Read the model definition and answer for the solid it produces. Units are mm, in the model's axes. Coordinates: 2 decimals unless noted, no trailing zeros. Loops run counter-clockwise (first coordinate to the right, second up) from the corner with the lowest first, then second, coordinate; pieces in that order, holes last. Notation, with made-up numbers: M 72.25,-7.5 L 101.25,-7.5 A29 cw 101.25,12.5 Z; hole C -32.75,-21 d3. An arc over 180 degrees is marked long. One line per item, written item: value. Start each with the question number.
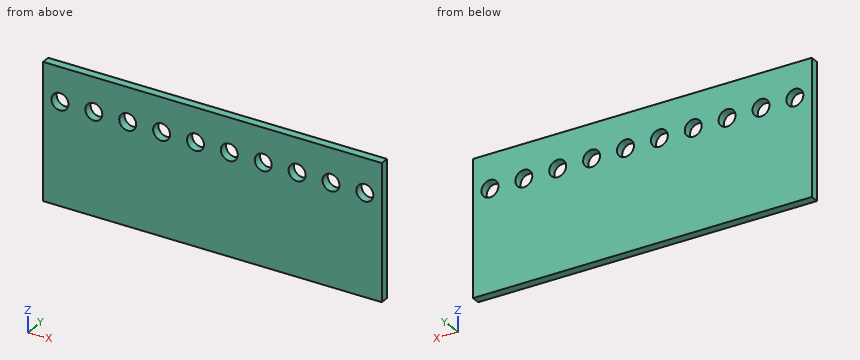
Autodesk Inventor part; units mm, degrees
ref_plane "YZ Plane" through (0, 0, 0) normal (1, 0, 0) x (0, 1, 0)
ref_plane "XZ Plane" through (0, 0, 0) normal (0, 1, 0) x (-1, 0, 0)
ref_plane "XY Plane" through (0, 0, 0) normal (0, 0, 1) x (1, 0, 0)
sketch "Sketch1" plane through (0, 0, 0) normal (0, 1, 0) x (-1, 0, 0)
  line L0 (127, 50.8) -> (-127, 50.8)
  line L1 (-127, 50.8) -> (-127, -50.8)
  line L2 (-127, -50.8) -> (127, -50.8)
  line L3 (127, -50.8) -> (127, 50.8)
  line L4 (127, 50.8) -> (-127, -50.8) construction
  line L5 (-127, 50.8) -> (127, -50.8) construction
  point P0 (0, 0)
  dimension "d3" = 101.6
  dimension "d13" = 254
extrude "Extrusion1" add sketch "Sketch1" against normal blind 6.35
sketch "Sketch3" plane through (0, 0, 0) normal (0, 1, 0) x (1, 0, 0)
  line L0 (-127, -50.8) -> (-127, 50.8) construction
  line L1 (-127, -25.4) -> (127, -25.4) construction
  line L2 (127, 50.8) -> (127, -50.8) construction
  line L3 (127, 50.8) -> (-127, 50.8) construction
  circle A0 centre (-114.3, -25.4) radius 6.35
  circle A1 centre (-88.9, -25.4) radius 6.35
  circle A2 centre (-63.5, -25.4) radius 6.35
  circle A3 centre (-38.1, -25.4) radius 6.35
  circle A4 centre (-12.7, -25.4) radius 6.35
  circle A5 centre (12.7, -25.4) radius 6.35
  circle A6 centre (38.1, -25.4) radius 6.35
  circle A7 centre (63.5, -25.4) radius 6.35
  circle A8 centre (88.9, -25.4) radius 6.35
  circle A9 centre (114.3, -25.4) radius 6.35
  point P0 (0, 0)
  dimension "d2" = 76.2
  dimension "d4" = 12.7
  dimension "d5" = 12.7
  dimension "d8" = 25.4
extrude "Extrusion2" cut sketch "Sketch3" against normal through all
properties part number "10-holes"
1) Consider line 1 along Z through (x, y) = (63.5, -5); line 2 along Z through (x, y) = (43, -2.5). Determine where each line is inside the solid, lowest interval first.
2) Section A-A (x = 63.5) is taken. Determine the outline of the cut face in (y, z), then the cut area to 3 significant figures.
3) Section B-B (y = -2) is taken. Count the separate pieces of the cut face and the enclosed holes in it, then the cut area to 3 significant figures.
4) A flat-ended cylindrical pin translates along its axis: pin 1 (7.5 mm diameter, centred on x = -12.7, z = 25.4, fed in from -Y). Find the tip coordinate at first contact, or state that the pin passes through.
Results found:
1. line 1: z = -50.8 to 19.05, 31.75 to 50.8
1. line 2: z = -50.8 to 21.36, 29.44 to 50.8
2. outline: M -6.35,-50.8 L 0,-50.8 L 0,19.05 L -6.35,19.05 Z; M -6.35,31.75 L 0,31.75 L 0,50.8 L -6.35,50.8 Z
2. area: 565 mm²
3. separate pieces: 1
3. enclosed holes: 10
3. area: 24,500 mm²
4. pin 1: passes through
